Autodesk Inventor part; units mm, degrees
ref_plane "YZ Plane" through (0, 0, 0) normal (1, 0, 0) x (0, 1, 0)
ref_plane "XZ Plane" through (0, 0, 0) normal (0, 1, 0) x (-1, 0, 0)
ref_plane "XY Plane" through (0, 0, 0) normal (0, 0, 1) x (1, 0, 0)
sketch "Boceto1" plane through (0, 0, 0) normal (0, 1, 0) x (-1, 0, 0)
  line L0 (0, 0) -> (-58, 0)
  line L1 (-58, 0) -> (-58, -55)
  line L2 (-58, -55) -> (0, -55)
  line L3 (0, -55) -> (0, 0)
  line L4 (0, -55) -> (-58, -55)
  dimension "d0" = 58
  dimension "d1" = 55
extrude "Extrusión1" add sketch "Boceto1" along normal blind 1.5
sketch "Boceto3" plane through (0, 0, 0) normal (0, 0, 1) x (1, 0, 0)
  line L0 (0, 1.5) -> (58, 1.5)
  line L1 (58, 1.5) -> (0, 1.5)
  line L2 (0, 1.5) -> (0, -40.5)
  line L3 (0, -40.5) -> (58, -40.5)
  line L4 (58, -40.5) -> (58, 1.5)
  point P0 (0, 0)
  dimension "d8" = 58
  dimension "d9" = 42
sketch "Boceto4" plane through (58, 0, -55) normal (0, 0, -1) x (-1, 0, 0)
  line L0 (58, 1.5) -> (0, 1.5)
  line L1 (0, 1.5) -> (58, 1.5)
  line L2 (58, 1.5) -> (58, -40.5)
  line L3 (58, -40.5) -> (0, -40.5)
  line L4 (0, -40.5) -> (0, 1.5)
  point P0 (58, 0)
  dimension "d10" = 42
extrude "Extrusión2" add sketch "Boceto4" against normal blind 1.5
extrude "Extrusión3" add sketch "Boceto3" against normal blind 1.5
sketch "Boceto6" plane through (0, -40.5, 0) normal (0, -1, 0) x (1, 0, 0)
  line L0 (58, 0) -> (58, -1.5)
  line L1 (58, -1.5) -> (0, -1.5)
  line L2 (58, -1.5) -> (0, -1.5)
  line L3 (0, -1.5) -> (0, -16.5)
  line L4 (0, -16.5) -> (58, -16.5)
  line L5 (58, -16.5) -> (58, -1.5)
  line L6 (58, -55) -> (0, -55)
  line L7 (58, -40) -> (58, -55)
  line L8 (0, -53.5) -> (58, -53.5)
  line L9 (58, -53.5) -> (58, -38.5)
  line L10 (58, -38.5) -> (0, -38.5)
  line L11 (0, -38.5) -> (0, -53.5)
  point P0 (0, 0)
  dimension "d17" = 15
  dimension "d50" = 15
  dimension "d51" = 58
  dimension "d61" = 58
  dimension "d62" = 15
extrude "Extrusión4" add sketch "Boceto6" against normal blind 1.5
sketch "Boceto7" plane through (0, -40.5, 0) normal (0, -1, 0) x (1, 0, 0)
  line L0 (58, 0) -> (58, -16.5)
  line L1 (0, 0) -> (0, -16.5)
  line L2 (58, -55) -> (58, -38.5)
  circle A0 centre (43.5, -8.25) radius 2
  circle A1 centre (14.5, -8.25) radius 2
  line L3 (0, -53.5) -> (0, -38.5)
  line L4 (0, -46) -> (58, -46)
  line L5 (58, -38.5) -> (58, -53.5)
  circle A2 centre (43.5, -46) radius 2
  circle A3 centre (14.5, -46) radius 2
  point P0 (58, -40)
  dimension "d23" = 4
  dimension "d25" = 4
  dimension "d63" = 4
  dimension "d64" = 4
extrude "Extrusión5" cut sketch "Boceto7" against normal blind 1.5
sketch "Boceto8" plane through (0, 1.5, 0) normal (0, 1, 0) x (1, 0, 0)
  line L0 (58, 0) -> (58, 55)
  line L1 (58, 1.5) -> (58, 53.5)
  line L2 (58, 45) -> (51, 45)
  circle A0 centre (51, 45) radius 2.25
  circle A1 centre (51, 10) radius 2.25
  circle A2 centre (4, 9) radius 2.25
  circle A3 centre (4, 46) radius 2.25
  circle A4 centre (29, 12) radius 2.25
  circle A5 centre (29, 43) radius 2.25
  point P0 (0, 0)
  point P1 (0, 55)
  dimension "d32" = 7
  dimension "d33" = 4.5
  dimension "d34" = 4.5
  dimension "d39" = 4.5
  dimension "d40" = 4.5
  dimension "d45" = 4.5
  dimension "d47" = 4.5
extrude "Extrusión7" cut sketch "Boceto8" against normal blind 1.5
fillet "Empalme1" radius 0.5 4 edges at (29, 1.5, -55) (29, -40.5, -55) (29, -40.5, 0) (29, 1.5, 0)
properties part number "suport motor"
The model under review builds one solid part; all positions refer to its coordinate system, in mm. A direction names the side the tool comes from. Round coordinates to 2 decimals unless told otherwise and drop trailing zeros. Order: outer loops, then holes, each group sorted by start corner. A loop starts at its lowest first (then second) coordinate and runs counter-clockwise, first axis right, second up.
Item 1: Add section A-A, the plane x = 51. State the section outline as (y, z) points, and give its area (3 significant figures).
Working result:
outline: (-40.5, -54.5) arc R0.5 ccw to (-40, -55) - (1, -55) arc R0.5 ccw to (1.5, -54.5) - (1.5, -47.25) - (0, -47.25) - (0, -53.5) - (-39, -53.5) - (-39, -38.5) - (-40.5, -38.5) - close; (-40.5, -16.5) - (-39, -16.5) - (-39, -1.5) - (0, -1.5) - (0, -7.75) - (1.5, -7.75) - (1.5, -0.5) arc R0.5 ccw to (1, 0) - (-40, 0) arc R0.5 ccw to (-40.5, -0.5) - close; (0, -42.75) - (1.5, -42.75) - (1.5, -12.25) - (0, -12.25) - close
area: 235 mm2
Item 2: Draft analysis for pull direction Z (two halves, no side actions). For faces 1 (the flat face through (29, -20, 0)), 2 (the flat face through (29, 1.5, -27)), 3 (the cylindrical face through (48.752, 0.76, -10.099)), 4 (the flat face through (29, -20, -55)), state which applies: released by +Z, released by -Z, zero draft, split by the parting line, or undercut.
Working result:
face 1: released by +Z
face 2: zero draft
face 3: undercut
face 4: released by -Z
Item 3: Add section B-B, the plane z = -15. State the section outline as (x, y) points, and give its area (3 significant figures).
Working result:
outline: (0, -40.5) - (58, -40.5) - (58, -39) - (0, -39) - close; (0, 0) - (58, 0) - (58, 1.5) - (0, 1.5) - close
area: 174 mm2
Item 4: Machinability: for faces 5 (the flat face through (29, -19, -1.5)), 6 (the cylindrical face through (13.026, -39.76, -6.898)), 7 (the cylindrical face through (49.34, 0.76, -46.52)), which of the approach directions +Z, -Z, +X, -X, +Y, -Y give a long, thin tool a straight path to every point of the face, cutting with its end or side? Answer none if there is none.
Working result:
face 5: +X, -X
face 6: -Y
face 7: +Y
Item 5: For pin 1 (1.5 mm diameter, centred on x = 48, z = -33, fed in from -Y), flat-tipped, find the tip position at first contact; note if it passes through.
Working result:
pin 1: stops at y = 0
Item 6: Add section D-D, the plane x = 21. State the section outline as (y, z) points.
Working result:
outline: (-40.5, -54.5) arc R0.5 ccw to (-40, -55) - (1, -55) arc R0.5 ccw to (1.5, -54.5) - (1.5, -0.5) arc R0.5 ccw to (1, 0) - (-40, 0) arc R0.5 ccw to (-40.5, -0.5) - (-40.5, -16.5) - (-39, -16.5) - (-39, -1.5) - (0, -1.5) - (0, -53.5) - (-39, -53.5) - (-39, -38.5) - (-40.5, -38.5) - close
Item 7: To check wall thickness, follow probe 1 along Z at (x, y) = (51, 1.1); probe 2 along Z at (x, y) = (43.5, -39.65); probe 3 along Z at (x, y) = (29, 0.75). State the ranges of each line that lie inside material, in increasing order.
Working result:
probe 1: z = -54.99 to -47.25, -42.75 to -12.25, -7.75 to -0.01
probe 2: z = -55 to -48, -44 to -38.5, -16.5 to -10.25, -6.25 to 0
probe 3: z = -55 to -45.25, -40.75 to -14.25, -9.75 to 0
Item 8: Add section C-C, the plane y = -15. State the section outline as (x, z) points.
Working result:
outline: (0, -55) - (58, -55) - (58, -53.5) - (0, -53.5) - close; (0, -1.5) - (58, -1.5) - (58, 0) - (0, 0) - close
